```python
from build123d import *

# Parameters (mm, degrees)
SKIZZE1_W                       = 260
SKIZZE1_H                       = 200
SKIZZE1_R                       = 1.749999999999997
SKIZZE1_R_2                     = 1.7500000000000038
SKIZZE1_R_3                     = 1.7500000000000042
AUFSATZ_LINEAR_AUSTRAGEN1_DEPTH = 8
SKIZZE2_R                       = 50
SCHNITT_LINEAR_AUSTRAGEN1_DEPTH = 8
SCHNITT_LINEAR_AUSTRAGEN4_DEPTH = 165.2071862008481
SCHNITT_LINEAR_AUSTRAGEN5_DEPTH = 4
VERRUNDUNG1_R                   = 2.3


with BuildPart() as part:
    # Skizze1 → Aufsatz-Linear austragen1 (new body)
    with BuildSketch(Plane(origin=(0, 0, 0), x_dir=(1, 0, 0), z_dir=(0, 1, 0))):
        Rectangle(SKIZZE1_W, SKIZZE1_H)
        with Locations(Location((-53, -92, 0), (0, 0, 270))):
            Circle(SKIZZE1_R, mode=Mode.SUBTRACT)
        with Locations(Location((53, -92, 0), (0, 0, 270))):
            Circle(SKIZZE1_R_2, mode=Mode.SUBTRACT)
        with Locations(Location((0, -92, 0), (0, 0, 270))):
            Circle(SKIZZE1_R_3, mode=Mode.SUBTRACT)
        with Locations(Location((-5.551e-14, 91.99999999999991, 0), (0, 0, 90))):
            Circle(SKIZZE1_R_3, mode=Mode.SUBTRACT)
        with Locations(Location((52.99999999999994, 91.99999999999991, 0), (0, 0, 90))):
            Circle(SKIZZE1_R_2, mode=Mode.SUBTRACT)
        with Locations(Location((-53.00000000000003, 91.99999999999989, 0), (0, 0, 90))):
            Circle(SKIZZE1_R, mode=Mode.SUBTRACT)
    extrude(amount=AUFSATZ_LINEAR_AUSTRAGEN1_DEPTH)

    # Skizze2 → Schnitt-Linear austragen1 (cut)
    with BuildSketch(Plane(origin=(0, 8, 0), x_dir=(1, 0, 0), z_dir=(0, 1, 0))):
        with Locations(Location((0, 0, 0), (0, 0, 270))):
            Circle(SKIZZE2_R)
    extrude(amount=-SCHNITT_LINEAR_AUSTRAGEN1_DEPTH, mode=Mode.SUBTRACT)

    # Skizze3 → Schnitt-Linear austragen4 (cut, through all)
    with BuildSketch(Plane.XZ):
        with BuildLine():
            ThreePointArc((60.00000000000001, 0), (59.947803224682126, 2.5021767593021864), (59.79130371550694, 5.000000000000675))
            Line((59.791303715506885, 5), (49.749371855331, 5))
            ThreePointArc((49.749371855331006, 5.000000000000001), (49.937303655516644, 2.503138752990944), (50.00000000000001, 0))
            ThreePointArc((50.00000000000001, -1.225e-14), (49.937303655516644, -2.503138752990955), (49.749371855331006, -5.00000000000001))
            Line((49.749371855331, -5), (59.791303715506885, -5))
            ThreePointArc((59.79130371550694, -5.0000000000006795), (59.947803224682126, -2.5021767593021957), (60.00000000000001, -1.47e-14))
        make_face()
        with BuildLine():
            ThreePointArc((59.79130371550694, 5.000000000000675), (57.257520364495285, 17.932550340356187), (51.961524227066455, 29.99999999999978))
            Line((51.961524227066455, 29.99999999999978), (43.30127018922205, 24.999999999999826))
            ThreePointArc((43.301270189222045, 24.999999999999822), (47.58787131429482, 15.342571615414302), (49.749371855331006, 5.000000000000001))
            Line((49.749371855331, 5), (59.791303715506885, 5))
        make_face()
        with BuildLine():
            Line((59.791303715506885, -5), (49.749371855331, -5))
            ThreePointArc((49.749371855331006, -5.00000000000001), (47.58787131429479, -15.342571615414398), (43.301270189221945, -24.999999999999986))
            Line((43.301270189221945, -24.999999999999993), (51.961524227066334, -29.999999999999993))
            ThreePointArc((51.961524227066334, -29.999999999999982), (57.25752036449525, -17.932550340356304), (59.79130371550694, -5.0000000000006795))
        make_face()
        with BuildLine():
            Line((-43.30127018922192, -25.00000000000002), (-51.961524227066306, -30.00000000000003))
            ThreePointArc((-51.96152422706632, -30.00000000000001), (-30.000000000000117, -51.961524227066256), (-2.7748e-13, -60.00000000000001))
            Line((-2.4633e-13, -60.00000000000001), (-1.9949e-13, -50.00000000000001))
            ThreePointArc((-1.8682e-13, -50.00000000000001), (-25.000000000000064, -43.3012701892219), (-43.30127018922194, -25.00000000000001))
        make_face()
        with BuildLine():
            ThreePointArc((3.67e-15, 60.00000000000001), (-29.999999999999876, 51.9615242270664), (-51.961524227066185, 30.000000000000256))
            Line((-51.961524227066185, 30.000000000000245), (-43.30127018922183, 25.0000000000002))
            ThreePointArc((-43.30127018922182, 25.000000000000213), (-24.999999999999897, 43.301270189221995), (3.06e-15, 50.00000000000001))
            Line((0, 50), (0, 60.00000000000001))
        make_face()
    extrude(amount=-SCHNITT_LINEAR_AUSTRAGEN4_DEPTH, mode=Mode.SUBTRACT)

    # Skizze3<5> → Schnitt-Linear austragen5 (cut)
    with BuildSketch(Plane.XZ):
        with BuildLine():
            Line((70.25062814466901, 5), (59.791303715506885, 5))
            ThreePointArc((59.79130371550694, 5.000000000000675), (59.947803224682126, 2.5021767593021864), (60.00000000000001, 0))
            ThreePointArc((60.00000000000001, -1.47e-14), (59.947803224682126, -2.5021767593021957), (59.79130371550694, -5.0000000000006795))
            Line((59.791303715506885, -5), (70.25062814466901, -5))
            Line((70.25062814466901, -5), (70.25062814466901, 5))
        make_face()
        with BuildLine():
            ThreePointArc((-59.79130371550711, -4.999999999998586), (-60.00000000000001, 7.35e-15), (-59.79130371550711, 4.999999999998601))
            Line((-59.791303715507226, 5), (-70.25062814466901, 5))
            Line((-70.25062814466901, 5), (-70.25062814466901, -5))
            Line((-70.25062814466901, -5), (-59.791303715507226, -5))
        make_face()
        with BuildLine():
            Line((-49.749371855331, -5), (-59.791303715507226, -5))
            ThreePointArc((-59.79130371550711, -4.999999999998586), (-57.257520364495555, -17.932550340355316), (-51.96152422706632, -30.00000000000001))
            Line((-51.961524227066306, -30.00000000000003), (-43.30127018922192, -25.00000000000002))
            ThreePointArc((-43.30127018922194, -25.00000000000001), (-47.58787131429479, -15.342571615414402), (-49.749371855331006, -4.999999999999992))
        make_face()
        with BuildLine():
            Line((-49.749371855331, 5), (-59.791303715507226, 5))
            ThreePointArc((-59.79130371550711, 4.999999999998601), (-60.00000000000001, 7.35e-15), (-59.79130371550711, -4.999999999998586))
            Line((-59.791303715507226, -5), (-49.749371855331, -5))
            ThreePointArc((-49.749371855331006, -4.999999999999992), (-50.00000000000001, 6.12e-15), (-49.749371855331006, 5.000000000000004))
        make_face()
        with BuildLine():
            Line((-43.30127018922183, 25.0000000000002), (-51.961524227066185, 30.000000000000245))
            ThreePointArc((-51.961524227066185, 30.000000000000256), (-57.25752036449551, 17.932550340355455), (-59.79130371550711, 4.999999999998601))
            Line((-59.791303715507226, 5), (-49.749371855331, 5))
            ThreePointArc((-49.749371855331006, 5.000000000000004), (-47.58787131429475, 15.342571615414519), (-43.30127018922182, 25.000000000000213))
        make_face()
        with BuildLine():
            ThreePointArc((51.961524227066455, 29.99999999999978), (30.00000000000011, 51.96152422706626), (3.67e-15, 60.00000000000001))
            Line((0, 60.00000000000001), (0, 50))
            ThreePointArc((3.06e-15, 50.00000000000001), (25.000000000000092, 43.30127018922189), (43.301270189222045, 24.99999999999982))
            Line((43.30127018922205, 24.999999999999826), (51.961524227066455, 29.99999999999978))
        make_face()
        with BuildLine():
            Line((-1.9949e-13, -50.00000000000001), (-2.4633e-13, -60.00000000000001))
            ThreePointArc((-2.7748e-13, -60.00000000000001), (29.99999999999987, -51.9615242270664), (51.961524227066334, -29.999999999999982))
            Line((51.961524227066334, -29.999999999999993), (43.301270189221945, -24.999999999999993))
            ThreePointArc((43.301270189221945, -24.999999999999986), (24.999999999999932, -43.30127018922198), (-1.8682e-13, -50.00000000000001))
        make_face()
    extrude(amount=-SCHNITT_LINEAR_AUSTRAGEN5_DEPTH, mode=Mode.SUBTRACT)

    # Verrundung1
    # the kernel refuses this fillet: 2.3 mm, written as the material it adds along each edge
    with BuildSketch(Plane(origin=(70.25062814466901, 0, 5), x_dir=(0, 0, -1), z_dir=(0, 1, 0))) as verrundung1_piece_1:
        with BuildLine():
            CenterArc((VERRUNDUNG1_R, VERRUNDUNG1_R), VERRUNDUNG1_R, 180, 90)
            Line((-8.9e-16, VERRUNDUNG1_R), (0, 0))
            Line((0, 0), (VERRUNDUNG1_R, 0))
        make_face()
    extrude(amount=4)
    with BuildSketch(Plane(origin=(70.25062814466901, 0, -5), x_dir=(-1, 0, 0), z_dir=(0, 1, 0))) as verrundung1_piece_2:
        with BuildLine():
            CenterArc((VERRUNDUNG1_R, VERRUNDUNG1_R), VERRUNDUNG1_R, 180, 90)
            Line((0, VERRUNDUNG1_R), (0, 0))
            Line((0, 0), (VERRUNDUNG1_R, 0))
        make_face()
    extrude(amount=4)
    with BuildSketch(Plane(origin=(-70.25062814466901, 0, -5), x_dir=(1, 0, 0), z_dir=(0, 1, 0))) as verrundung1_piece_3:
        with BuildLine():
            CenterArc((VERRUNDUNG1_R, -VERRUNDUNG1_R), VERRUNDUNG1_R, 90, 89.99999999999997)
            Line((0, -VERRUNDUNG1_R), (0, 0))
            Line((0, 0), (VERRUNDUNG1_R, 0))
        make_face()
    extrude(amount=4)
    with BuildSketch(Plane(origin=(-70.25062814466901, 0, 5), x_dir=(0, 0, -1), z_dir=(0, 1, 0))) as verrundung1_piece_4:
        with BuildLine():
            CenterArc((VERRUNDUNG1_R, -VERRUNDUNG1_R), VERRUNDUNG1_R, 90, 90)
            Line((0, -VERRUNDUNG1_R), (0, 0))
            Line((0, 0), (VERRUNDUNG1_R, 0))
        make_face()
    extrude(amount=4)
    with BuildSketch(Plane(origin=(51.96152422706646, 4, 29.99999999999978), x_dir=(0.48263674044551186, 0, -0.8758206304787137), z_dir=(0, 1, 0))) as verrundung1_piece_5:
        with BuildLine():
            CenterArc((2.346306800066914, 2.2995429563643968), VERRUNDUNG1_R, 178.8577537601654, 92.2844924796575)
            Line((0.04676384370252609, 2.345392621956658), (0, 0))
            ThreePointArc((0, 0), (1.1960782328293844, -0.01192287745045764), (2.392156465658705, -7e-17))
        make_face()
    extrude(amount=4)
    with BuildSketch(Plane(origin=(51.961524227066334, 4, -29.99999999999999), x_dir=(-0.8660254037844398, 0, 0.499999999999998), z_dir=(0, 1, 0))) as verrundung1_piece_6:
        with BuildLine():
            CenterArc((2.345858778401576, 2.2999999999999994), VERRUNDUNG1_R, 177.71550752035841, 92.2844924796417)
            ThreePointArc((0.04768677130146285, 2.3916811091852797), (0.011922877450426, 1.1960782328291542), (0, 0))
            Line((0, 0), (2.34585877840158, -4e-17))
        make_face()
    extrude(amount=4)
    with BuildSketch(Plane(origin=(-51.96152422706631, 4, -30.00000000000002), x_dir=(0.8660254037844404, 0, 0.49999999999999717), z_dir=(0, 1, 0))) as verrundung1_piece_7:
        with BuildLine():
            CenterArc((2.3458587784015195, 2.2999999999999994), VERRUNDUNG1_R, 177.71550752035327, 92.28449247964659)
            ThreePointArc((0.04768677130141288, 2.3916811091854857), (0.01192287745041601, 1.196078232829249), (0, 0))
            Line((0, 0), (2.3458587784015132, -4e-17))
        make_face()
    extrude(amount=4)
    with BuildSketch(Plane(origin=(-2.6083e-13, 4, -60), x_dir=(1.086e-14, 0, 1), z_dir=(0, 1, 0))) as verrundung1_piece_8:
        with BuildLine():
            CenterArc((2.3458587784010057, -2.3), VERRUNDUNG1_R, 89.99999999999973, 92.28449247964573)
            ThreePointArc((0.04768677130089817, -2.3916811091854364), (0.01192287745039645, -1.1960782328292843), (0, 0))
            Line((0, 0), (2.3458587784010163, 0))
        make_face()
    extrude(amount=4)
    with BuildSketch(Plane(origin=(1.84e-15, 4, 60.00000000000001), x_dir=(-7.8e-16, 0, -1), z_dir=(0, 1, 0))) as verrundung1_piece_9:
        with BuildLine():
            CenterArc((2.3458587784015865, 2.3), VERRUNDUNG1_R, 177.71550752035446, 92.28449247964545)
            ThreePointArc((0.04768677130148023, 2.3916811091854395), (0.011922877450453, 1.1960782328292412), (0, 0))
            Line((0, 0), (2.3458587784015847, 0))
        make_face()
    extrude(amount=4)
    with BuildSketch(Plane(origin=(-51.961524227066185, 4, 30.00000000000025), x_dir=(0.8660254037844354, 0, -0.5000000000000054), z_dir=(0, 1, 0))) as verrundung1_piece_10:
        with BuildLine():
            CenterArc((2.3458587784015092, -2.3), VERRUNDUNG1_R, 90, 92.28449247965011)
            ThreePointArc((0.04768677130141038, -2.3916811091856207), (0.0119228774504358, -1.1960782328293367), (0, 0))
            Line((0, 0), (2.3458587784015092, -2e-16))
        make_face()
    extrude(amount=4)


solid = part.part
```
Geometry check sheet. Reference: the model listing, model coordinates, mm. A direction names the side the tool comes from. Coordinates: 2 decimals unless noted, no trailing zeros. Order: outer loops, then holes, each group sorted by start corner. A loop starts at its lowest first (then second) coordinate and runs counter-clockwise, first axis right, second up.
Item 1: Section check D-D (y = 6). Enter the section's corners in (x, z).
Item 2: Section check A-A (x = 64.5). Enter the section's corners in (y, z), plus the area to 3 significant figures.
Item 3: Scan lines: line 1 along X through (y, z) = (5.25, 92); line 2 along X through (y, z) = (1.25, 5.5); line 3 along X through (y, z) = (2, 90.5). Record each from-to range of solid material in increasing order.
Item 4: Tool access check on faces 5 (the cylindrical face through (-50, 6, 0)), 6 (the flat face through (25, 4, 46)), 7 (the flat face through (130, 4, 1)). Record the directions out of +Z, -Z, +X, -X, +Y, -Y that give a thin tool (end or side, any length) a straight path to the whole face; none if there is none.
Item 5: Depth check by flat-ended pin: pin 1 (10.5 mm diameter, centred on x = 23.5, z = -42, fed in from -Y). Enter the tip coordinate at first touch or a pass-through.
Item 6: Section check C-C (x = -19). Enter the section's corners in (y, z), plus the area to 3 significant figures.
Item 7: Mould release check, pull along X, two halves, no side actions. Record for faces 1 (the cylindrical face through (25.317, 6.028, -43.117)), 2 (the flat face through (-2, 4, -100)), 3 (the cylindrical face through (24.682, 6.028, 43.483)), 4 (the flat face through (-130, 4, 1)): released by +X, released by -X, zero draft, split by the parting line, or undercut.
Item 8: Section check B-B (z = -21.5). Enter the section's corners in (x, y).
Check sheet entries:
1. outline: (-130, -100) - (130, -100) - (130, 100) - (-130, 100) - close; hole circle Ø3.5 at (-53, -92); hole circle Ø3.5 at (-53, 92); hole (-50.72, -32.05) arc R60 ccw to (-2.39, -59.95) arc R2.3 ccw to (0, -57.65) - (0, -50) arc R50 ccw to (43.3, -25) - (49.93, -28.83) arc R2.3 ccw to (53.12, -27.9) arc R60 ccw to (53.12, 27.9) arc R2.3 ccw to (49.93, 28.83) - (43.3, 25) arc R50 ccw to (0, 50) - (0, 57.65) arc R2.3 ccw to (-2.39, 59.95) arc R60 ccw to (-50.72, 32.05) arc R2.3 ccw to (-49.93, 28.83) - (-43.3, 25) arc R50 ccw to (-43.3, -25) - (-49.93, -28.83) arc R2.3 ccw to start; hole circle Ø3.5 at (0, -92); hole circle Ø3.5 at (0, 92); hole circle Ø3.5 at (53, -92); hole circle Ø3.5 at (53, 92)
2. outline: (0, -100) - (8, -100) - (8, 100) - (0, 100) - (0, 5) - (4, 5) - (4, -5) - (0, -5) - close
2. area: 1,560 mm2
3. line 1: x = -130 to -54.75, -51.25 to -1.75, 1.75 to 51.25, 54.75 to 130
3. line 2: x = -130 to -59.75, 59.75 to 130
3. line 3: x = -130 to -53.9, -52.1 to -0.9, 0.9 to 52.1, 53.9 to 130
4. face 5: +Y, -Y
4. face 6: -Y
4. face 7: +Z, -Z, +X, +Y, -Y
5. pin 1: stops at y = 4
6. outline: (0, -100) - (8, -100) - (8, -56.91) - (0, -56.91) - close; (0, 56.91) - (8, 56.91) - (8, 100) - (0, 100) - close
6. area: 689 mm2
7. face 1: undercut
7. face 2: zero draft
7. face 3: undercut
7. face 4: released by -X
8. outline: (-130, 0) - (-56.02, 0) - (-56.02, 4) - (-45.14, 4) - (-45.14, 8) - (-130, 8) - close; (56.02, 0) - (130, 0) - (130, 8) - (56.02, 8) - close
